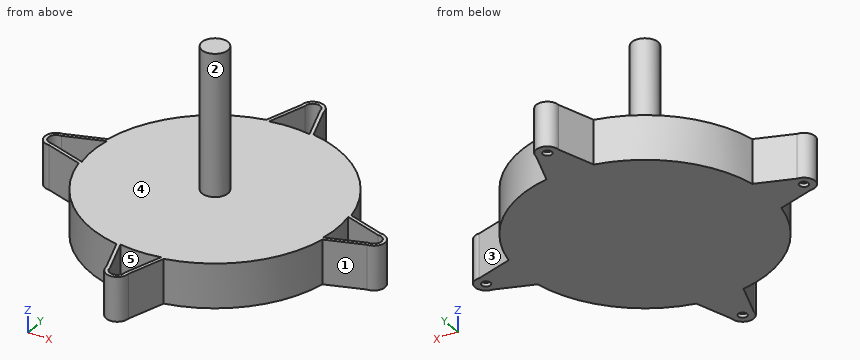
from build123d import *

# Parameters (mm, degrees)
SKETCH1_R           = 70
BOSS_EXTRUDE1_DEPTH = 25
BOSS_EXTRUDE3_DEPTH = 25
CUT_EXTRUDE1_DEPTH  = 23
CUT_EXTRUDE2_REACH  = 122.942
SKETCH6_R           = 2.5
CIRPATTERN2_COUNT   = 4
SKETCH7_R           = 7.375
BOSS_EXTRUDE4_DEPTH = 80


with BuildPart() as part:
    # Sketch1 → Boss-Extrude1 (new body)
    with BuildSketch(Plane.XY):
        Circle(SKETCH1_R)
    extrude(amount=BOSS_EXTRUDE1_DEPTH)

    # Sketch3 → Boss-Extrude3 (add)
    with BuildSketch(Plane.XY):
        with BuildLine():
            Line((13.329299006, 68.719209745), (6.292622314, 89.613315607))
            ThreePointArc((6.292622314, 89.613315607), (0, 95.90593792), (-6.292622314, 89.613315607))
            Line((-6.292622314, 89.613315607), (-13.329299006, 68.719209745))
            ThreePointArc((-13.329299006, 68.719209745), (0, 70), (13.329299006, 68.719209745))
        make_face()
    boss_extrude3 = extrude(amount=BOSS_EXTRUDE3_DEPTH)

    # Sketch5 → Cut-Extrude1 (cut)
    with BuildSketch(Plane.XY.offset(25)):
        with BuildLine():
            Line((11.433900255, 68.080881008), (4.282324573, 89.316158104))
            ThreePointArc((4.282324573, 89.316158104), (0, 93.90593792), (-4.282324573, 89.316158104))
            Line((-4.282324573, 89.316158104), (-11.433900255, 68.080881008))
            ThreePointArc((-11.433900255, 68.080881008), (0, 69.180406265), (11.433900255, 68.080881008))
        make_face()
    cut_extrude1 = extrude(amount=-CUT_EXTRUDE1_DEPTH, mode=Mode.SUBTRACT)

    # Sketch6 → Cut-Extrude2 (cut, up to next)
    with BuildSketch(Plane.XY.offset(2), mode=Mode.PRIVATE) as cut_extrude2_sk1:
        with Locations((0, 89.613315607)):
            Circle(SKETCH6_R)
    cut_extrude2_tool1 = extrude(cut_extrude2_sk1.sketch, amount=-CUT_EXTRUDE2_REACH, mode=Mode.PRIVATE) & part.part
    cut_extrude2 = cut_extrude2_tool1.solids().sort_by_distance((0, 89.613316, 2))[0]
    add(cut_extrude2, mode=Mode.SUBTRACT)

    # CirPattern2: Boss-Extrude3, Cut-Extrude1, Cut-Extrude2 ×4 about axis
    cirpattern2_axis = Axis((0, 0, 0), (0, 0, 1))
    add([boss_extrude3.rotate(cirpattern2_axis, i * 360 / CIRPATTERN2_COUNT) for i in range(1, CIRPATTERN2_COUNT)])
    add([cut_extrude1.rotate(cirpattern2_axis, i * 360 / CIRPATTERN2_COUNT) for i in range(1, CIRPATTERN2_COUNT)], mode=Mode.SUBTRACT)
    add([cut_extrude2.rotate(cirpattern2_axis, i * 360 / CIRPATTERN2_COUNT) for i in range(1, CIRPATTERN2_COUNT)], mode=Mode.SUBTRACT)

    # Sketch7 → Boss-Extrude4 (add)
    with BuildSketch(Plane.XY.offset(25)):
        Circle(SKETCH7_R)
    extrude(amount=BOSS_EXTRUDE4_DEPTH)


solid = part.part
The listing builds one solid part. Answer for the finished solid, in the listing's coordinates (mm). Face numbers are marked on the shaded views. A direction names the side the tool comes from. Give positions to 0.01 mm unless a question says otherwise; leave off trailing zeros. Write each loop counter-clockwise with the first axis right and the second up, starting at its lowest first coordinate (ties: lowest second). Pieces come first, ordered by that corner, then holes. Notation, with made-up numbers: (-9.75, 34) - (2.25, 34) arc R12 ccw to (2.25, 56) - close; hole circle Ø3 at (-19, 2.25). An arc over 180 degrees is marked (long way). Use a Markdown table: item, result.
1. Section A-A on x = 0 is taken. Write down the section's boundary in (y, z) (3 decimals), plus the area to 3 significant figures.
Values follow:
| item | result |
|---|---|
| outline | (-95.906, 0) - (-92.113, 0) - (-92.113, 2) - (-93.906, 2) - (-93.906, 25) - (-95.906, 25) - close; (-87.113, 0) - (87.113, 0) - (87.113, 2) - (69.18, 2) - (69.18, 25) - (7.375, 25) - (7.375, 105) - (-7.375, 105) - (-7.375, 25) - (-69.18, 25) - (-69.18, 2) - (-87.113, 2) - close; (92.113, 0) - (95.906, 0) - (95.906, 25) - (93.906, 25) - (93.906, 2) - (92.113, 2) - close |
| area | 4,820 mm² |
2. Each of these flat-tipped pins is pushed along its axis until it touches: P1, Ø8, axis at x = -89.61, y = 0, coming from the +Z side; P2, Ø11.5, axis at x = -81, y = -3.5, coming from the +Z side; P3, Ø5, axis at x = -47.5, z = 18, coming from the +Y side. Where does it stop, or does it pass through?
Values follow:
| item | result |
|---|---|
| P1 | stops at z = 2 |
| P2 | stops at z = 25 |
| P3 | stops at y = 53.62 |
3. Section C-C on z = 83.5 is taken. Write down the section's boundary in (x, y) (3 decimals).
Values follow:
| item | result |
|---|---|
| outline | circle Ø14.75 at (0, 0) |
4. Find the intervals of material crossed by probe 1 along Y at (x, z) = (0, 0.85); probe 2 along Z at (x, y) = (-25.5, 5), in increasing order. Write a range as from..to.
Values follow:
| item | result |
|---|---|
| probe 1 | y = -95.91..-92.11, -87.11..87.11, 92.11..95.91 |
| probe 2 | z = 0..25 |
5. For a pull along X with two mould halves and no side action, classify the marked faces 3, 4 and 5 as released by +X, released by -X, zero draft, split by the parting line, or undercut.
Values follow:
| item | result |
|---|---|
| face 3 | released by +X |
| face 4 | zero draft |
| face 5 | undercut |
6. A tool of negligible diameter and unlimited length cuts with its end or side. For the marked faces 1 and 2, from which of +Z, -Z, +X, -X, +Y, -Y can it reach the whole face along a straight path? Write none if from no direction.
Values follow:
| item | result |
|---|---|
| face 1 | +Z, -Z, +X, -Y |
| face 2 | +Z |
7. Section D-D on y = 80 is taken. Write down the section's boundary in (x, z).
Values follow:
| item | result |
|---|---|
| outline | (-9.53, 0) - (9.53, 0) - (9.53, 25) - (7.42, 25) - (7.42, 2) - (-7.42, 2) - (-7.42, 25) - (-9.53, 25) - close |
